CAD build for the part. Positions are in the model's coordinates, mm. A direction names the side the tool comes from. Coordinates: 2 decimals unless noted, no trailing zeros. Loops run counter-clockwise (first coordinate to the right, second up) from the corner with the lowest first, then second, coordinate; pieces in that order, holes last. Notation, with made-up numbers: (11, -24) -> (22, -24) arc R20 ccw to (22, -10) -> close; hole circle Ø2 at (7.25, 79.5). An arc over 180 degrees is marked (long way). Answer as CSV lines item,"result". Start each with the question number.
Autodesk Inventor part; units mm, degrees
ref_plane "Work Plane1" through (133, -30, -66) normal (0, 0, -1) x (-1, 0, 0)
ref_plane "YZ Plane" through (0, 0, 0) normal (1, 0, 0) x (0, 1, 0)
ref_plane "XZ Plane" through (0, 0, 0) normal (0, 1, 0) x (-1, 0, 0)
sketch "Sketch1" plane through (0, 0, 0) normal (0, 0, 1) x (1, 0, 0)
  line L0 (-36, 36) -> (36, 36)
  line L1 (36, 36) -> (36, -36)
  line L2 (36, -36) -> (-36, -36)
  line L3 (-36, -36) -> (-36, 36)
  point P0 (0, 0)
  dimension "d0" = 72
  dimension "d1" = 36
  dimension "d2" = 72
  dimension "d3" = 36
extrude "Plate1" add sketch "Sketch1" along normal blind 6
sketch "Sketch2" plane through (-36, -30, 6) normal (0, -1, 0) x (1, 0, 0)
  line L0 (72, 0) -> (0, 0)
  line L1 (0, 0) -> (0, -72)
  line L2 (0, -72) -> (72, -72)
  line L3 (72, -72) -> (72, 0)
edge flange "Flange1" height 72 angle 90 thickness 6 bend radius 6 thickness toward (0, -1, 0) relief tear relief width 6 relief depth 3 edges at (0, -36, 0) wall of the first edge with corners at (36, -30, 6) (-36, -30, 6) (-36, -30, -66) (36, -30, -66)
bend "Bend1"
corner "Corner1"
sketch "Sketch3" plane through (-36, -30, -66) normal (0, 1, 0) x (1, 0, 0)
  line L0 (72, -60) -> (72, 0)
  line L1 (72, 0) -> (181, 0)
  line L2 (181, 0) -> (181, -60)
  line L3 (181, -60) -> (72, -60)
  line L4 (72, -60) -> (72, 0)
  point P0 (36, -66)
  dimension "d15" = 109
  dimension "d16" = 60
sheet face with bend "Face2" sketch "Sketch3" thickness 6 toward (0, -1, 0) bend radius 6
bend "Bend2"
sketch "Sketch4" plane through (139, -36, -66) normal (1, 0, 0) x (0, 1, 0)
  line L0 (0, 60) -> (0, 0)
  line L1 (0, 0) -> (100.6, 0)
  line L2 (100.6, 0) -> (100.6, 60)
  line L3 (100.6, 60) -> (0, 60)
edge flange "Flange2" height 100.6 angle 90 thickness 6 bend radius 6 thickness toward (1, 0, 0) relief tear relief width 6 relief depth 3 edges at (145, -30, -36) wall of the first edge with corners at (139, -36, -6) (139, -36, -66) (139, 64.6, -66) (139, 64.6, -6)
bend "Bend3"
corner "Corner2"
sketch "Sketch5" plane through (145, 64.6, -6) normal (1, 0, 0) x (0, 0, -1)
  circle A0 centre (30, -30) radius 25
  line L0 (60, 0) -> (60, -88.6)
  line L1 (0, -88.6) -> (0, 0)
  line L2 (0, 0) -> (60, 0)
  point P0 (-6, -64.6)
  point P1 (55, -30)
  point P2 (5, -30)
  dimension "d32" = 60
  dimension "d33" = 30
  dimension "d34" = 30
  dimension "d35" = 50
  dimension "d36" = 30
  dimension "d37" = 30
hole "Hole1" at (145, 34.6, -11) at (145, 34.6, -61) direction (-1, 0, 0) diameter 5 end through all
sketch "Sketch6" plane through (0, 0, 6) normal (0, 0, 1) x (1, 0, 0)
  circle A0 centre (0, 0) radius 12.7
  line L0 (36, -36) -> (-36, -36)
  circle A1 centre (0, 0) radius 33.5
  line L1 (0, 0) -> (29.0119, -16.75)
  line L2 (0, 0) -> (-29.0119, -16.75)
  line L3 (0, 0) -> (0, 33.5)
  point P0 (0, 0)
  point P1 (0, 12.7)
  point P2 (10.9985, -6.35)
  point P3 (-10.9985, -6.35)
  dimension "d45" = 36
  dimension "d46" = 25.4
  dimension "d47" = 67
  dimension "d48" = 120
  dimension "d49" = 120
  dimension "d50" = 0
hole "Hole2" at (0, 12.7, 6) at (-10.9985, -6.35, 6) at (10.9985, -6.35, 6) at (29.0119, -16.75, 6) at (-29.0119, -16.75, 6) direction (0, 0, -1) diameter 5 end through all
sketch "Sketch7" plane through (-36, -30, -6) normal (0, 1, 0) x (1, 0, 0)
  line L0 (169, 60) -> (0, 60)
  line L1 (169, 0) -> (72, 0)
  line L2 (0, 0) -> (0, 60)
  line L3 (72, 0) -> (72, 20)
  point P0 (36, -6)
  point P1 (121.5202, 30)
  point P2 (36, 30)
  point P3 (36, 10)
  dimension "d65" = 60
  dimension "d66" = 72
  dimension "d67" = 30
  dimension "d68" = 30
  dimension "d69" = 36
  dimension "d70" = 20
  dimension "d71" = 10
  dimension "d72" = 36
  dimension "d73" = 99.0404
  dimension "d74" = 49.5202
hole "Hole3" at (85.5202, -30, -36) at (0, -30, -36) at (0, -30, -16) direction (0, -1, 0) diameter 5 end through all
mirror "Mirror1" about plane through (139, -24, -66) normal (0, 0, -1)
ref_plane "Work Plane1" through (133, -30, -66) normal (0, 0, -1) x (-1, 0, 0)
split "Split1" plane through (133, -30, -66) removes the side toward (0, 0, 1)
equation "\"d2\" = d0"
equation "\"d33\" = 0.5 * d32"
equation "\"d34\" = d33"
equation "\"d36\" = d34"
equation "\"d37\" = d36"
equation "\"d43\" = Thickness"
equation "\"d49\" = d48"
equation "\"d56\" = Thickness"
equation "\"d63\" = Thickness"
equation "\"d4\" = Thickness"
equation "\"d5\" = BendReliefWidth"
equation "\"d6\" = BendReliefDepth"
equation "\"d7\" = MinimumRemnant"
equation "\"d8\" = TransitionRadius"
equation "\"d11\" = BendRadius"
equation "\"d12\" = CornerReliefSize"
equation "\"d13\" = GapSize"
equation "\"d14\" = JacobiRadiusSize"
equation "\"d17\" = BendRadius"
equation "\"d18\" = BendReliefWidth"
equation "\"d20\" = MinimumRemnant"
equation "\"d19\" = BendReliefDepth"
equation "\"d21\" = TransitionRadius"
equation "\"d22\" = BendReliefWidth"
equation "\"d23\" = BendReliefDepth"
equation "\"d24\" = MinimumRemnant"
equation "\"d25\" = TransitionRadius"
equation "\"d28\" = BendRadius"
equation "\"d29\" = CornerReliefSize"
equation "\"d30\" = GapSize"
equation "\"d31\" = JacobiRadiusSize"
equation "\"BendRadius\" = Thickness"
equation "\"BendReliefWidth\" = Thickness"
equation "\"BendReliefDepth\" = 0.5 * Thickness"
equation "\"CornerReliefSize\" = 4 * Thickness"
equation "\"MinimumRemnant\" = 2 * Thickness"
equation "\"TransitionRadius\" = BendRadius"
equation "\"JacobiRadiusSize\" = BendRadius"
equation "\"GapSize\" = Thickness"
properties part number "motorHolder" material "Steel, Mild"
Item 1: Wall check: probe 1 along X at (y, z) = (-16.75, -134.6); probe 2 along X at (y, z) = (-6, -133); probe 3 along Z at (x, y) = (0, -34.5). Give the ranges that are in metal, low to high.
Item 2: Which spindle directions (+Z, -Z, +X, -X, +Y, -Y) get a long thin tool onto all of the face, cutting with end or side? Do faces 4 (the face through (47, -30, -96)), 5 (the face through (81, -31, -66)), 6 (the face through (1, 36, -135)), 7 (the face through (139, 20, -96)), 8 (the face through (106.4, -30.2, -126)). Say none if no direction does.
Item 3: Flat gauge pins, fed straight in: pin 1 Ø4 at (x, z) = (0, -96) entering from +Y; pin 2 Ø3.5 at (y, z) = (-5.5, -130.5) entering from +X; pin 3 Ø6.5 at (x, y) = (-11, -6.35) entering from +Z; pin 4 Ø1.8 at (x, z) = (16.5, -134.5) entering from +Y. Where does each tip first touch, or does it go through?
Item 4: Saw through at C-C (z = -121). Write the cut outline in (x, y).
Item 5: Saw through at D-D (y = -16.75). Write the cut outline in (x, z).
Item 6: Saw through at A-A (z = -96). Write the cut outline in (x, y), plus the area to 3 significant figures.
Item 7: Two-plate mould, pull along Y, no slides. Class faces 1 (the face through (47, -36, -96)), 2 (the face through (29.122, -14.252, -134.958)), 3 (the face through (-0.504, -28.196, -130.289)): pulls with the +Y half, pulls with the -Y half, needs draft (parallel to the pull), parting line crosses it, or undercut.
Item 8: Saw through at B-B (y = 21.5). Write the cut outline in (x, z), plus the area to 3 significant figures.
Geometry check:
1,probe 1,"-36 to -31.51, -26.51 to 26.51, 31.51 to 36"
1,probe 2,"-36 to -13.47, -8.52 to 8.52, 13.47 to 36"
1,probe 3,"-131.81 to -118.5, -113.5 to -98.5, -93.5 to -66"
2,face 4,"+Z, -X, +Y"
2,face 5,"+Z, +X, -X, +Y, -Y"
2,face 6,"+Z, -Z, +X, -X, +Y"
2,face 7,"+Z, -Z, -X, +Y"
2,face 8,"-Z, +X, +Y, -Y"
3,pin 1,"through"
3,pin 2,"x = 36"
3,pin 3,"z = -132"
3,pin 4,"y = 36"
4,outline,"(-36, -36) -> (133, -36) arc R12 ccw to (145, -24) -> (145, 32.1) -> (139, 32.1) -> (139, -24) arc R6 cw to (133, -30) -> (-36, -30) -> close; (139, 37.1) -> (145, 37.1) -> (145, 64.6) -> (139, 64.6) -> close"
5,outline,"(-36, -138) -> (-31.51, -138) -> (-31.51, -132) -> (-36, -132) -> close; (-26.51, -138) -> (26.51, -138) -> (26.51, -132) -> (-26.51, -132) -> close; (31.51, -138) -> (36, -138) -> (36, -132) -> (31.51, -132) -> close; (139, -126) -> (145, -126) -> (145, -66) -> (139, -66) -> close"
6,outline,"(-36, -36) -> (-2.5, -36) -> (-2.5, -30) -> (-36, -30) -> close; (2.5, -36) -> (83.02, -36) -> (83.02, -30) -> (2.5, -30) -> close; (88.02, -36) -> (133, -36) arc R12 ccw to (145, -24) -> (145, 64.6) -> (139, 64.6) -> (139, -24) arc R6 cw to (133, -30) -> (88.02, -30) -> close"
6,area,"1,570 mm2"
7,face 1,"pulls with the -Y half"
7,face 2,"undercut"
7,face 3,"pulls with the +Y half"
8,outline,"(-36, -138) -> (36, -138) -> (36, -132) -> (-36, -132) -> close; (139, -126) -> (145, -126) -> (145, -66) -> (139, -66) -> close"
8,area,"792 mm2"
